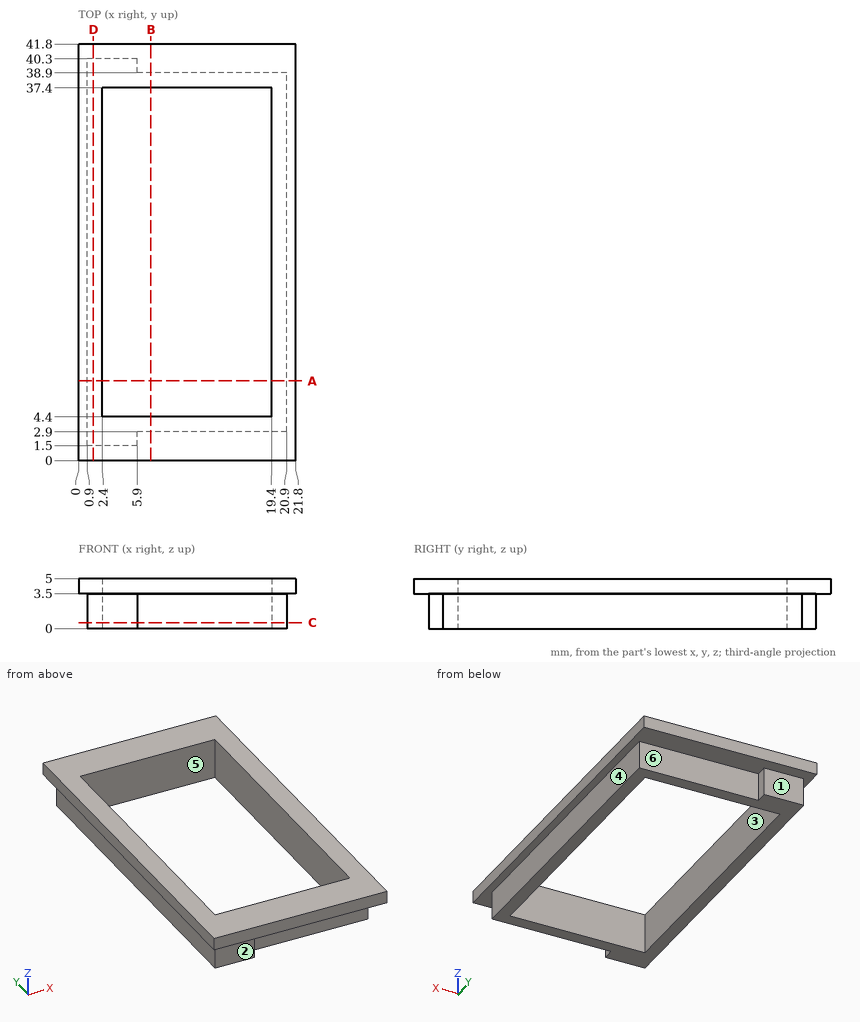
Geometry check sheet. Reference: drawing and pictorial views, mm from the part's lowest x, y, z. A direction names the side the tool comes from. Coordinates: 2 decimals unless noted, no trailing zeros. Order: outer loops, then holes, each group sorted by start corner. A loop starts at its lowest first (then second) coordinate and runs counter-clockwise, first axis right, second up. Notation, with made-up numbers: (69.5, 43) - (121.5, 43) arc R17 ccw to (121.5, 74) - close; hole circle Ø10 at (-36, 23). An arc over 180 degrees is marked (long way). One line per item, written item: value.
(1) Sectioned sample at A-A (y = 8). Enter the section's corners in (x, z).
Data:
outline: (0, 3.5) - (0.9, 3.5) - (0.9, 0) - (2.4, 0) - (2.4, 5) - (0, 5) - close; (19.4, 0) - (20.9, 0) - (20.9, 3.5) - (21.8, 3.5) - (21.8, 5) - (19.4, 5) - close
(2) Sectioned sample at B-B (x = 7.25). Enter the section's corners in (y, z).
Data:
outline: (0, 3.5) - (2.9, 3.5) - (2.9, 0) - (4.4, 0) - (4.4, 5) - (0, 5) - close; (37.4, 0) - (38.9, 0) - (38.9, 3.5) - (41.8, 3.5) - (41.8, 5) - (37.4, 5) - close
(3) Sectioned sample at D-D (x = 1.5). Enter the section's corners in (y, z), and give its area (4 significant figures).
Data:
outline: (0, 3.5) - (1.5, 3.5) - (1.5, 0) - (40.3, 0) - (40.3, 3.5) - (41.8, 3.5) - (41.8, 5) - (0, 5) - close
area: 198.5 mm^2
(4) Access from +Z, -Z, +X, -X, +Y, -Y to the whole of each face (thin tool, end or side, straight path). Record for the marked faces 1, 2 and 3.
Data:
face 1: -Z, +X, -X, +Y
face 2: -Z, +X, -X, -Y
face 3: +Z, -Z
(5) Thickness scan on probe 1 along X at (y, z) = (15, 1.95); probe 2 along Y at (x, z) = (11.25, 4.1); probe 3 along Y at (x, z) = (17.5, 1.9). Record the ranges inside material, lowest first. Write a range as from..to.
Data:
probe 1: x = 0.9..2.4, 19.4..20.9
probe 2: y = 0..4.4, 37.4..41.8
probe 3: y = 2.9..4.4, 37.4..38.9
(6) Release check for a two-part mould opening along X. For the marked faces 4, 5 and 6 record: +X half, -X half, draft (parallel to the pull), parting line (faces both ways), or undercut.
Data:
face 4: +X half
face 5: undercut
face 6: draft
(7) Sectioned sample at C-C (z = 0.6). Enter the section's corners in (x, y).
Data:
outline: (0.9, 1.5) - (5.9, 1.5) - (5.9, 2.9) - (20.9, 2.9) - (20.9, 38.9) - (5.9, 38.9) - (5.9, 40.3) - (0.9, 40.3) - close; hole (2.4, 4.4) - (19.4, 4.4) - (19.4, 37.4) - (2.4, 37.4) - close
(8) Depth check by flat-ended pin: pin 1 Ø1.1 at (x, z) = (3, 1.5) entering from -Y; pin 2 Ø3 at (y, z) = (28.5, 1.5) entering from -X; pin 3 Ø0.7 at (y, z) = (39.5, 1.5) entering from +X; pin 4 Ø8 at (x, y) = (10, 10.5) entering from -Z. Enter the tip coordinate at first touch or a pass-through.
Data:
pin 1: stops at y = 1.5
pin 2: stops at x = 0.9
pin 3: stops at x = 5.9
pin 4: passes through
